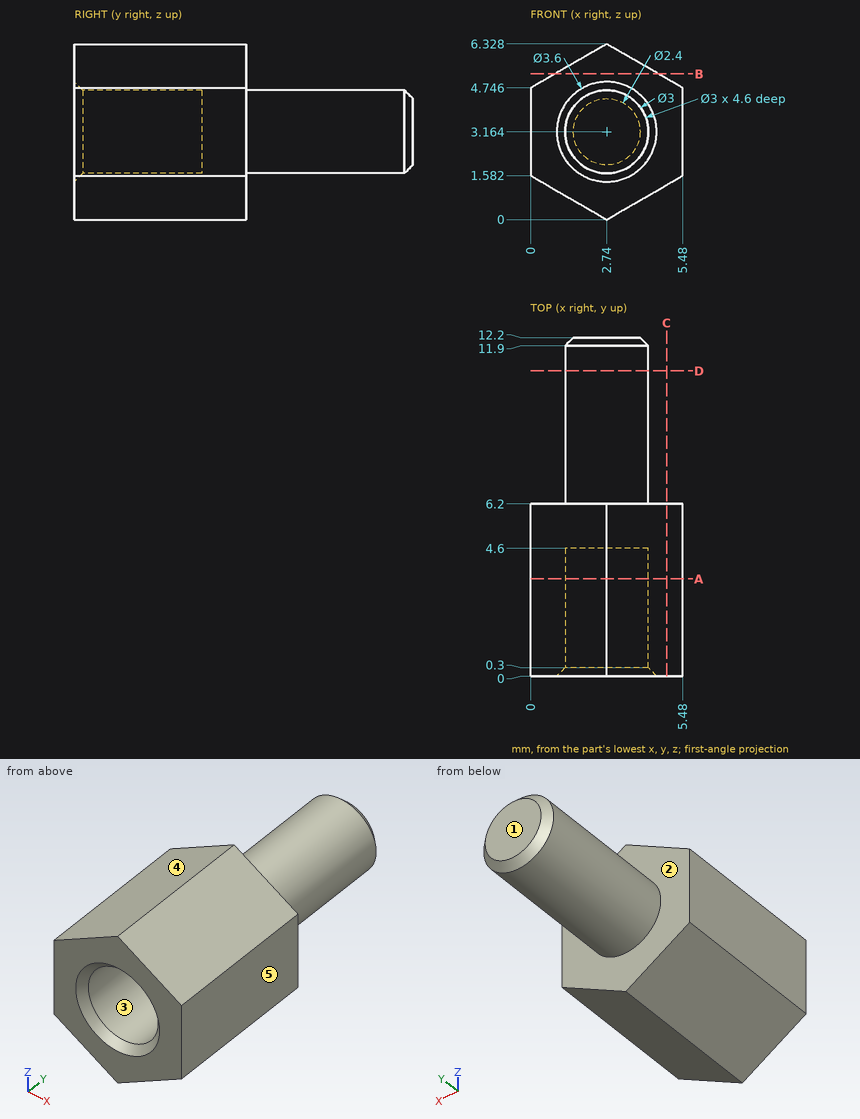
Verification items for this drawing (mm, ordinates from the low corner). A direction names the side the tool comes from. Round coordinates to 2 decimals unless told otherwise and drop trailing zeros. Write each loop counter-clockwise with the first axis right and the second up, starting at its lowest first coordinate (ties: lowest second). Pieces come first, ordered by that corner, then holes. Notation, with made-up numbers: (-4, -39.5) - (5, -39.5) arc R25 cw to (5, -0.5) - close; hole circle Ø4 at (55, -34). An arc over 180 degrees is marked (long way). Answer as a JSON object with one key per item and string values. Group by question number.
Q1. Section check C-C, the plane x = 4.9. Enter the section's corners in (y, z).
Q2. Section check A-A, the plane y = 3.5. Enter the section's corners in (x, z).
Q3. Section check D-D, the plane y = 11. Enter the section's corners in (x, z).
Q4. Section check B-B, the plane z = 5.25. Enter the section's corners in (x, y).
Q5. Thickness scan on line 1 (X direction, y = 3.5, z = 3.25); line 2 (Y direction, x = 3.45, z = 2.25); line 3 (Y direction, x = 5, z = 4). Record the ranges inside material, lowest first.
Q6. Tool access check on the marked faces 1 and 2. Record the directions out of +Z, -Z, +X, -X, +Y, -Y that give a thin tool (end or side, any length) a straight path to the whole face; none if there is none.
Q7. Mould release check, pull along Z, two halves, no side actions. Record for the marked faces 3, 4 and 5: released by +Z, released by -Z, zero draft, split by the parting line, or undercut.
Q8. Go/stop test with flat-tipped pins: pin 1 Ø0.9 at (x, z) = (2, 3) entering from -Y; pin 2 Ø2 at (x, y) = (2.5, 5.5) entering from -Z. Record where each tip stops, or that it passes through.
Found:
{
 "1": {"outline": "(0, 1.25) - (6.2, 1.25) - (6.2, 5.08) - (0, 5.08) - close"},
 "2": {"outline": "(0, 1.58) - (2.74, 0) - (5.48, 1.58) - (5.48, 4.75) - (2.74, 6.33) - (0, 4.75) - close; hole circle Ø3 at (2.74, 3.16)"},
 "3": {"outline": "circle Ø3 at (2.74, 3.16)"},
 "4": {"outline": "(0.87, 0) - (4.61, 0) - (4.61, 6.2) - (0.87, 6.2) - close"},
 "5": {"line 1": "x = 0 to 1.24, 4.24 to 5.48", "line 2": "y = 4.6 to 12.2", "line 3": "y = 0 to 6.2"},
 "6": {"face 1": "+Z, -Z, +X, -X, +Y", "face 2": "+Y"},
 "7": {"face 3": "undercut", "face 4": "released by +Z", "face 5": "zero draft"},
 "8": {"pin 1": "stops at y = 4.6", "pin 2": "stops at z = 0"}
}
